Build history of the part. All positions in model axes, mm. Face numbers are marked on the shaded views. A direction names the side the tool comes from. Give positions to 0.01 mm unless a question says otherwise; leave off trailing zeros. Loops run counter-clockwise (first coordinate to the right, second up) from the corner with the lowest first, then second, coordinate; pieces in that order, holes last. Notation, with made-up numbers: (-18.75, 6) -> (11.25, 6) arc R30 ccw to (11.25, 33) -> close; hole circle Ø5 at (-21.5, -21). An arc over 180 degrees is marked (long way). One line per question, with ' | ' between items. Start each with the question number.
(1) 3-axis set-ups, long thin cutter, end or side, ignore diameter. For the marked faces 1, 2 and 3: which of +Z, -Z, +X, -X, +Y, -Y reach the whole face in a straight line?
(2) Drill centre lines: L1, parallel to Z at x = 26, y = 17; L2, parallel to Y at x = 26, z = -4.5; L3, parallel to Y at x = -15, z = -0.75. Where is each one in solid material? Low to high. Write a range as from..to.
(3) Slice it at C-C, the plane z = 0. Give the number of separate pieces and of enclosed holes in the cut face, then the cut area to 3 significant figures.
(4) Flat gauge pins, fed straight in: pin 1 Ø1.5 at (x, z) = (8, -0.5) entering from +Y; pin 2 Ø3 at (y, z) = (-26, 0) entering from +X; pin 3 Ø5 at (x, z) = (24, 0) entering from -Y; pin 4 Ø1.6 at (x, z) = (-19.5, 1.5) entering from -Y. Where does each tip first touch, or does it go through?
(5) Slice it at A-A, the plane x = 26. Write the cut outline in (y, z), then the cut area to 3 significant figures.
(6) Slice it at B-B, the plane z = 3.5. Write the cut outline in (x, y), then the cut area to 4 significant figures.
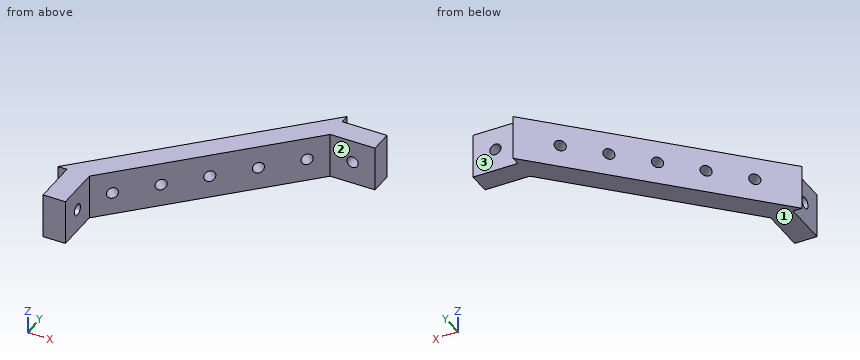
```python
from build123d import *

# Parameters (mm, degrees)
MAIN_DEPTH         = 5
SKETCH2_R          = 1.25
FIXHOLE1_DEPTH     = 43
SKETCH3_R          = 1.25
FIXHOLE2_DEPTH     = 43
SKETCH6_R          = 1.25
CUT_EXTRUDE2_DEPTH = 35.648232278
LPATTERN1_COUNT    = 5
LPATTERN1_PITCH    = 10


with BuildPart() as part:
    # Sketch1 → Main (new body, symmetric)
    with BuildSketch(Plane.XY):
        Polygon((-21, -21), (21, 21), (21, 19), (31, 19), (31, 14), (21, 14), (-14, -21), (-14, -31), (-19, -31), (-19, -21), align=None)
    extrude(amount=MAIN_DEPTH, both=True)

    # Sketch2 → FixHole1 (cut, through all)
    with BuildSketch(Plane(origin=(21, 0, 0), x_dir=(0, 0, -1), z_dir=(1, 0, 0))):
        with Locations((0, -26)):
            Circle(SKETCH2_R)
    extrude(amount=-FIXHOLE1_DEPTH, mode=Mode.SUBTRACT)

    # Sketch3 → FixHole2 (cut, through all)
    with BuildSketch(Plane(origin=(0, -21, 0), x_dir=(-1, 0, 0), z_dir=(0, -1, 0))):
        with Locations((-26, 0)):
            Circle(SKETCH3_R)
    extrude(amount=-FIXHOLE2_DEPTH, mode=Mode.SUBTRACT)

    # Sketch6 → Cut-Extrude2 (cut, through all)
    with BuildSketch(Plane(origin=(3.5, -3.5, 0), x_dir=(0, 0, 1), z_dir=(-0.707106781, 0.707106781, 0))):
        with Locations((0, 20)):
            Circle(SKETCH6_R)
    cut_extrude2 = extrude(amount=CUT_EXTRUDE2_DEPTH, mode=Mode.SUBTRACT)

    # LPattern1: Cut-Extrude2 ×5
    with Locations(*[Vector(-0.707106781, -0.707106781, 0) * (i * LPATTERN1_PITCH) for i in range(1, LPATTERN1_COUNT)]):
        add(cut_extrude2, mode=Mode.SUBTRACT)


solid = part.part
```
Final values:
1) face 1: -Z, +X, -X, +Y, -Y | face 2: +Z, -Z, +X, -Y | face 3: +Z, -Z, +X, +Y
2) L1: -5..-1.25, 1.25..5 | L2: 14..19 | L3: -31..-27, -25..-15
3) separate pieces: 8 | enclosed holes: 0 | area: 283 mm2
4) pin 1: y = 8.75 | pin 2: x = -14 | pin 3: y = 14 | pin 4: y = -31
5) outline: (14, -5) -> (19, -5) -> (19, -1.25) -> (14, -1.25) -> close; (14, 1.25) -> (19, 1.25) -> (19, 5) -> (14, 5) -> close | area: 37.5 mm2
6) outline: (-21, -21) -> (-19, -21) -> (-19, -31) -> (-14, -31) -> (-14, -21) -> (21, 14) -> (31, 14) -> (31, 19) -> (21, 19) -> (21, 21) -> close | area: 369.5 mm2
